Study the drawing (mm; zero at the part's minimum x, y, z) and answer. A direction names the side the tool comes from. Round coordinates to 2 decimals unless told otherwise and drop trailing zeros. Loops run counter-clockwise (first coordinate to the right, second up) from the corner with the lowest first, then second, coordinate; pieces in that order, holes last. Notation, with made-up numbers: M -30,12 L -26,12 A21 ccw -26,36 Z; hole C 43,11.5 d9. An arc over 180 degrees is marked long. Put each result on its own line as item: value. Start each with the question number.
(1) Section B-B, the plane z = 15.5 is taken. Determine the outline of the cut face in (x, y).
(2) Flat-ended cylindrical pins translate along their axes: P1, Ø1.5, axis at x = 30.5, z = 22.5, coming from the +Y side; P2, Ø2.5, axis at x = 26.1, y = 4.93, coming from the +Z side; P3, Ø4, axis at x = 27, z = 5, coming from the -Y side; P4, Ø4, axis at y = 11, z = 62, coming from the -X side. Find the tip coordinate at first contact, or state that the pin passes through.
(3) Section C-C, the plane y = 25.45 is taken. Determine the outline of the cut face in (x, z).
(4) Section A-A, the plane x = 18.35 is taken. Determine the outline of the cut face in (y, z).
(5) Which of the six approach directions +Z, -Z, +X, -X, +Y, -Y give full straight-line access (tool end or side, diameter ignored) to the marked faces 1, 2 and 3?
(6) Straight lines are drawn through the part: line 1 (Y direction, x = 10.6, z = 56.25) (1 decimal); line 2 (Z direction, x = 3, y = 17); line 3 (Z direction, x = 3, y = 22). For each, find the intervals that lie inside material, in ascending order.
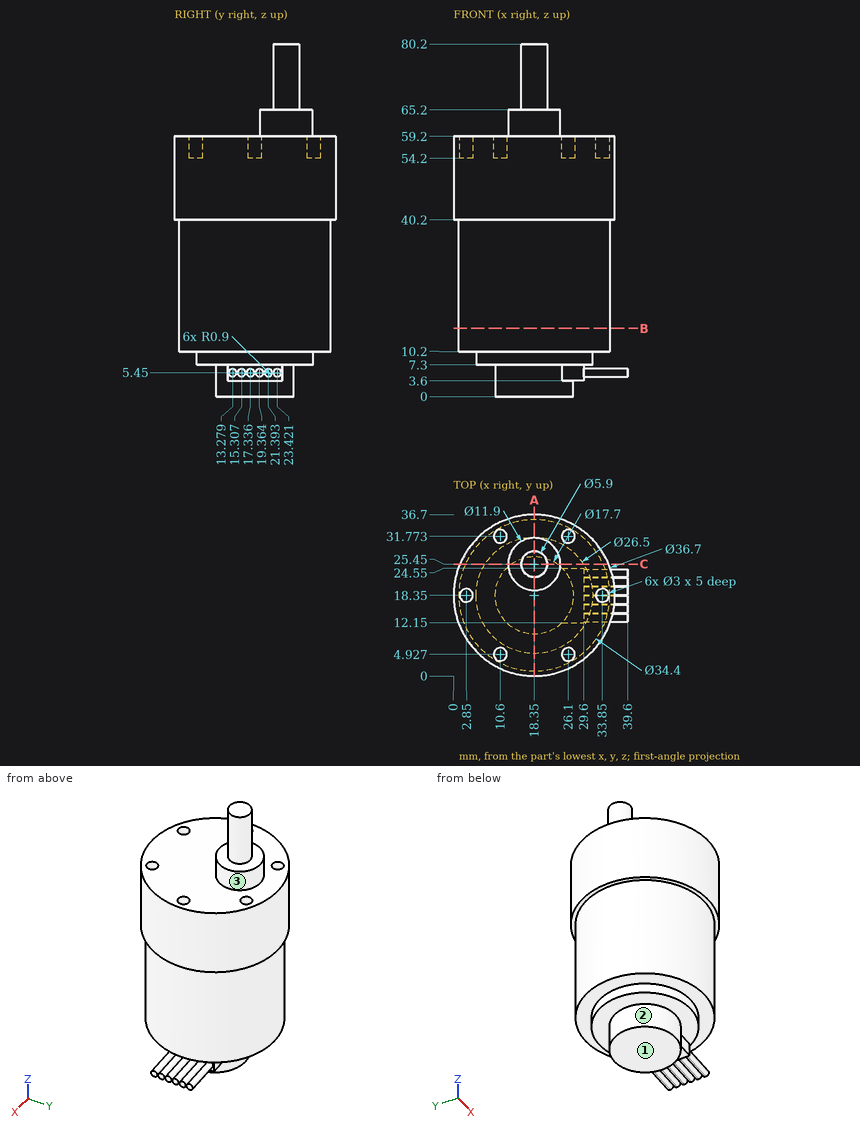
Recorded:
1. outline: C 18.35,18.35 d34.4
2. P1: stops at y = 31.23
2. P2: stops at z = 54.2
2. P3: stops at y = 12.15
2. P4: passes through
3. outline: M 1.43,40.2 L 2.68,40.2 L 2.68,10.2 L 7.16,10.2 L 7.16,7.3 L 13.07,7.3 L 13.07,0 L 23.63,0 L 23.63,7.3 L 29.54,7.3 L 29.54,10.2 L 34.02,10.2 L 34.02,40.2 L 35.27,40.2 L 35.27,59.2 L 24.3,59.2 L 24.3,65.2 L 21.3,65.2 L 21.3,80.2 L 15.4,80.2 L 15.4,65.2 L 12.4,65.2 L 12.4,59.2 L 1.43,59.2 Z
4. outline: M 0,40.2 L 1.15,40.2 L 1.15,10.2 L 5.1,10.2 L 5.1,7.3 L 9.5,7.3 L 9.5,0 L 27.2,0 L 27.2,7.3 L 31.6,7.3 L 31.6,10.2 L 35.55,10.2 L 35.55,40.2 L 36.7,40.2 L 36.7,59.2 L 31.4,59.2 L 31.4,65.2 L 28.4,65.2 L 28.4,80.2 L 22.5,80.2 L 22.5,65.2 L 19.5,65.2 L 19.5,59.2 L 0,59.2 Z
5. face 1: -Z, +X, -X, +Y, -Y
5. face 2: -Z
5. face 3: +Z
6. line 1: y = 1.7 to 3.4, 6.4 to 30.3, 33.3 to 35
6. line 2: z = 10.2 to 54.2
6. line 3: z = 10.2 to 59.2
